Can you work these out from the model? Positions are in its coordinate system, mm. A direction names the side the tool comes from. Give positions to 0.01 mm unless a question says otherwise; leave off trailing zeros. Write each loop counter-clockwise with the first axis right and the second up, starting at its lowest first coordinate (ties: lowest second). Pieces come first, ordered by that corner, then holes.
from build123d import *

# Parameters (mm, degrees)
F1_DEPTH  = 5
F3_DEPTH  = 40
F5_DEPTH  = 20
F7_DEPTH  = 16
F8_DEPTH  = 25
F10_DEPTH = 25


with BuildPart() as f1:
    # F0 (on Top) → F1 (new body)
    with BuildSketch(Plane.XY):
        Polygon((1.75, 20), (1.75, 10), (40, 10), (40, -10), (-40, -10), (-40, 10), (-1.75, 10), (-1.75, 20), (-50, 20), (-50, -20), (50, -20), (50, 20), align=None)
        Polygon((1.75, 10), (1.75, 4), (35, 4), (35, -4), (-35, -4), (-35, 4), (-1.75, 4), (-1.75, 10), (-40, 10), (-40, -10), (40, -10), (40, 10), align=None)
        Polygon((1.75, 3), (5.05, 3), (5.05, -3), (-5.05, -3), (-5.05, 3), (-1.75, 3), (-1.75, 4), (-35, 4), (-35, -4), (35, -4), (35, 4), (1.75, 4), align=None)
        with BuildLine():
            Line((5.05, -3), (5.05, 3))
            Line((5.05, 3), (1.75, 3))
            Line((1.75, 3), (1.75, 1.4142135624))
            ThreePointArc((1.75, 1.4142135624), (2.1213203436, 0.75), (2.25, 0))
            ThreePointArc((2.25, 0), (-0.75, -2.1213203436), (-1.75, 1.4142135624))
            Line((-1.75, 1.4142135624), (-1.75, 3))
            Line((-1.75, 3), (-5.05, 3))
            Line((-5.05, 3), (-5.05, -3))
            Line((-5.05, -3), (5.05, -3))
        make_face()
        with BuildLine():
            ThreePointArc((2.25, 0), (2.1213203436, 0.75), (1.75, 1.4142135624))
            ThreePointArc((1.75, 1.4142135624), (0, 2.25), (-1.75, 1.4142135624))
            ThreePointArc((-1.75, 1.4142135624), (-0.75, -2.1213203436), (2.25, 0))
        make_face()
    extrude(amount=F1_DEPTH)

    # F2 (on face) → F3 (join)
    with BuildSketch(Plane.XY.offset(5)):
        with BuildLine():
            Line((-40, 10), (-40, -10))
            Line((-40, -10), (40, -10))
            Line((40, -10), (40, 10))
            Line((40, 10), (1.75, 10))
            Line((1.75, 10), (1.75, 1.4142135624))
            ThreePointArc((1.75, 1.4142135624), (0, 2.25), (-1.75, 1.4142135624))
            Line((-1.75, 1.4142135624), (-1.75, 10))
            Line((-1.75, 10), (-40, 10))
        make_face()
    extrude(amount=F3_DEPTH)

    # F4 (on face) → F5 (cut)
    with BuildSketch(Plane.XY.offset(45)):
        with BuildLine():
            Line((-35, -4), (35, -4))
            Line((35, -4), (35, 4))
            Line((35, 4), (1.75, 4))
            Line((1.75, 4), (1.75, 1.4142135624))
            ThreePointArc((1.75, 1.4142135624), (0, 2.25), (-1.75, 1.4142135624))
            Line((-1.75, 1.4142135624), (-1.75, 4))
            Line((-1.75, 4), (-35, 4))
            Line((-35, 4), (-35, -4))
        make_face()
    extrude(amount=-F5_DEPTH, mode=Mode.SUBTRACT)

    # F6 (on face) → F7 (cut)
    with BuildSketch(Plane.XY.offset(25)):
        with BuildLine():
            Line((5.05, -3), (5.05, 3))
            Line((5.05, 3), (1.75, 3))
            Line((1.75, 3), (1.75, 1.4142135624))
            ThreePointArc((1.75, 1.4142135624), (2.1213203436, 0.75), (2.25, 0))
            ThreePointArc((2.25, 0), (-0.75, -2.1213203436), (-1.75, 1.4142135624))
            Line((-1.75, 1.4142135624), (-1.75, 3))
            Line((-1.75, 3), (-5.05, 3))
            Line((-5.05, 3), (-5.05, -3))
            Line((-5.05, -3), (5.05, -3))
        make_face()
    extrude(amount=-F7_DEPTH, mode=Mode.SUBTRACT)

    # F8 (cut): a face of the model
    f8_faces = [f1.faces().sort_by_distance(p)[0] for p in [
        (0, 0, 25),
    ]]
    extrude(f8_faces, amount=-F8_DEPTH, mode=Mode.SUBTRACT)

    # F9 (on face) → F10 (cut)
    with BuildSketch(Plane.XY.offset(25)):
        Polygon((-35, 20), (-35, 4), (-1.75, 4), (1.75, 4), (35, 4), (35, 20), (1.75, 20), (-1.75, 20), align=None)
    extrude(amount=F10_DEPTH, mode=Mode.SUBTRACT)


solid = f1.part
(1) Imagine slicing it at A-A, the plane z = 20. Write out the boundary of the cut face in (x, y).
Returned:
outline: (-40, -10) - (40, -10) - (40, 10) - (1.75, 10) - (1.75, 3) - (5.05, 3) - (5.05, -3) - (-5.05, -3) - (-5.05, 3) - (-1.75, 3) - (-1.75, 10) - (-40, 10) - close
(2) Imagine slicing it at C-C, the plane y = -5. Write out the boundary of the cut face in (x, z), plus the area to 3 significant figures.
Returned:
outline: (-50, 0) - (50, 0) - (50, 5) - (40, 5) - (40, 45) - (-40, 45) - (-40, 5) - (-50, 5) - close
area: 3,700 mm2
(3) For faces 1 (the face through (0, -3, 17)), 2 (the face through (35, 3, 35)), 3 (the face through (-40, 0, 25)), 4 (the face through (-21, 10, 16)), which set-ups out of +Z, -Z, +X, -X, +Y, -Y let a thin tool reach every point of the face, with its end or its side?
Returned:
face 1: +Z
face 2: +Z, +Y
face 3: +Z, -X, +Y, -Y
face 4: +Z, +X, -X, +Y
(4) If I drill on L1, parallel to X at y = 10.5, z = 4.5; L2, parallel to Z at x = -43, y = 15.5; L3, parallel to Z at x = 27, y = 8.5, over which ranges is the centre line in solid material (lowest first)?
Returned:
L1: x = -50 to -1.75, 1.75 to 50
L2: z = 0 to 5
L3: z = 0 to 25
(5) Will these pins go through, and if not, where does the flat tip stop? P1, Ø8, axis at x = 0, z = 10, coming from the +Y side; P2, Ø10, axis at y = -4, z = 26.5, coming from the +X side; P3, Ø5, axis at x = 12.5, z = 22, coming from the -Y side; P4, Ø2.5, axis at x = 0, y = 0, coming from the +Z side (1 decimal).
Returned:
P1: stops at y = 10
P2: stops at x = 40
P3: stops at y = -10
P4: passes through
(6) Imagine slicing it at B-B, the plane y = 9. Write out the boundary of the cut face in (x, z), plus the area to 3 significant figures.
Returned:
outline: (-50, 0) - (-1.75, 0) - (-1.75, 25) - (-35, 25) - (-35, 45) - (-40, 45) - (-40, 5) - (-50, 5) - close; (1.75, 0) - (50, 0) - (50, 5) - (40, 5) - (40, 45) - (35, 45) - (35, 25) - (1.75, 25) - close
area: 2,210 mm2
(7) If we mould it in two halves opening along X, with no side actions, what happens to faces 5 (the face through (1.75, 9, 10)), 6 (the face through (-9.4, -4.3, 45)), 7 (the face through (40, 0, 25))? For each: +X half, -X half, draft (parallel to the pull), parting line (faces both ways), or undercut.
Returned:
face 5: undercut
face 6: draft
face 7: +X half
(8) Imagine slicing it at D-D, the plane x = 0. Write out the boundary of the cut face in (y, z), plus the area to 3 significant figures.
Returned:
outline: (-20, 0) - (-2.25, 0) - (-2.25, 9) - (-3, 9) - (-3, 25) - (-4, 25) - (-4, 45) - (-10, 45) - (-10, 5) - (-20, 5) - close
area: 352 mm2
